The listing builds one solid part. Answer for the finished solid, in the listing's coordinates (mm). A direction names the side the tool comes from. Give positions to 0.01 mm unless a question says otherwise; leave off trailing zeros. Order: outer loops, then holes, each group sorted by start corner. A loop starts at its lowest first (then second) coordinate and runs counter-clockwise, first axis right, second up. Notation, with made-up numbers: (-4, 44) - (28, 44) arc R22 cw to (28, 76) - close; hole circle Ø11 at (-1.5, 73.5). An arc over 180 degrees is marked (long way). Answer in a Markdown table with one row per item.
from build123d import *

# Parameters (mm, degrees)
CROQUIS1_R              = 1.75
SALIENTE_EXTRUIR1_DEPTH = 3
CROQUIS3_W              = 6
CROQUIS3_H              = 30
CROQUIS3_R              = 1.75
SALIENTE_EXTRUIR4_DEPTH = 14
REDONDEO1_R             = 2


with BuildPart() as part:
    # Croquis1 → Saliente-Extruir1 (new body)
    # profile 1 of 2: a face of its own
    with BuildSketch(Plane.XY):
        Polygon((-24, 12.5), (24, 12.5), (24, 22.5), (24, 27.5), (-24, 27.5), (-24, 22.5), align=None)
        with Locations((-21, 25)):
            Circle(CROQUIS1_R, mode=Mode.SUBTRACT)
        with Locations((21, 25)):
            Circle(CROQUIS1_R, mode=Mode.SUBTRACT)
    # profile 2 of 2: a face of its own
    with BuildSketch(Plane.XY):
        Polygon((-24, -2.5), (24, -2.5), (24, 2.5), (24, 12.5), (-24, 12.5), (-24, 2.5), align=None)
        with Locations((-21, 0)):
            Circle(CROQUIS1_R, mode=Mode.SUBTRACT)
        with Locations((21, 0)):
            Circle(CROQUIS1_R, mode=Mode.SUBTRACT)
    extrude(amount=SALIENTE_EXTRUIR1_DEPTH)

    # Croquis3 → Saliente-Extruir4 (add)
    # profile 1 of 2: a face of its own
    with BuildSketch(Plane.XY.offset(3)):
        with Locations((-21, 12.5)):
            Rectangle(CROQUIS3_W, CROQUIS3_H)
        with Locations((-21, 0)):
            Circle(CROQUIS3_R, mode=Mode.SUBTRACT)
        with Locations((-21, 25)):
            Circle(CROQUIS3_R, mode=Mode.SUBTRACT)
    # profile 2 of 2: a face of its own
    with BuildSketch(Plane.XY.offset(3)):
        with Locations((21, 12.5)):
            Rectangle(CROQUIS3_W, CROQUIS3_H)
        with Locations((21, 0)):
            Circle(CROQUIS3_R, mode=Mode.SUBTRACT)
        with Locations((21, 25)):
            Circle(CROQUIS3_R, mode=Mode.SUBTRACT)
    extrude(amount=SALIENTE_EXTRUIR4_DEPTH)

    # Redondeo1
    # the kernel refuses this fillet: 2 mm, written as the material it takes off along each edge
    with BuildSketch(Plane(origin=(-24, 32.5, 0), x_dir=(1, 0, 0), z_dir=(0, -1, 0)), Plane(origin=(24, -7.5, 0), x_dir=(-1, 0, 0), z_dir=(0, 1, 0))) as redondeo1_piece_1:
        with BuildLine():
            CenterArc((REDONDEO1_R, REDONDEO1_R), REDONDEO1_R, 180, 90)
            Line((0, REDONDEO1_R), (0, 0))
            Line((0, 0), (REDONDEO1_R, 0))
        make_face()
    extrude(amount=40, mode=Mode.SUBTRACT)


solid = part.part
Item 1: Consider line 1 (X direction, y = 0, z = 5.25); line 2 (Y direction, x = 21, z = 12.25); line 3 (X direction, y = 5, z = 12.75). Determine where each line is inside the solid, lowest interval first.
Answer block:
| item | result |
|---|---|
| line 1 | -24 to -22.75, -19.25 to -18, 18 to 19.25, 22.75 to 24 |
| line 2 | -2.5 to -1.75, 1.75 to 23.25, 26.75 to 27.5 |
| line 3 | -24 to -18, 18 to 24 |
Item 2: Find section D-D on y = 19.5. Write down the section's boundary in (x, z), then the cut area to 3 significant figures.
Answer block:
| item | result |
|---|---|
| outline | (-24, 2) arc R2 ccw to (-22, 0) - (22, 0) arc R2 ccw to (24, 2) - (24, 17) - (18, 17) - (18, 3) - (-18, 3) - (-18, 17) - (-24, 17) - close |
| area | 310 mm² |
Item 3: Find section B-B on x = 21. Write down the section's boundary in (y, z).
Answer block:
| item | result |
|---|---|
| outline | (-2.5, 0) - (-1.75, 0) - (-1.75, 17) - (-2.5, 17) - close; (1.75, 0) - (23.25, 0) - (23.25, 17) - (1.75, 17) - close; (26.75, 0) - (27.5, 0) - (27.5, 17) - (26.75, 17) - close |
Item 4: Determine the mould class of faces 3 (the face through (-0.3, 27.5, 2.7)), 4 (the face through (23.43, 12.29, 0.6)), 5 (the face through (19.71, 26.18, 8.38)) for opening direction X: pulls with the +X half, pulls with the -X half, needs draft (parallel to the pull), parting line crosses it, or undercut.
Answer block:
| item | result |
|---|---|
| face 3 | needs draft |
| face 4 | pulls with the +X half |
| face 5 | undercut |
Item 5: This flat-tipped pin is pushed along its axis until it touches: P1, Ø3, axis at x = -21, y = 0, coming from the +Z side. Where does it stop, or does it pass through?
Answer block:
| item | result |
|---|---|
| P1 | through |
Item 6: Find section A-A on z = 12. Write down the section's boundary in (x, y).
Answer block:
| item | result |
|---|---|
| outline | (-24, -2.5) - (-18, -2.5) - (-18, 27.5) - (-24, 27.5) - close; (18, -2.5) - (24, -2.5) - (24, 27.5) - (18, 27.5) - close; hole circle Ø3.5 at (-21, 0); hole circle Ø3.5 at (-21, 25); hole circle Ø3.5 at (21, 0); hole circle Ø3.5 at (21, 25) |
Item 7: Find section C-C on y = 0. Write down the section's boundary in (x, z).
Answer block:
| item | result |
|---|---|
| outline | (-24, 2) arc R2 ccw to (-22.75, 0.15) - (-22.75, 17) - (-24, 17) - close; (-19.25, 0) - (19.25, 0) - (19.25, 17) - (18, 17) - (18, 3) - (-18, 3) - (-18, 17) - (-19.25, 17) - close; (22.75, 0.15) arc R2 ccw to (24, 2) - (24, 17) - (22.75, 17) - close |
Item 8: Which of the six approach directions +Z, -Z, +X, -X, +Y, -Y give full straight-line access (tool end or side, diameter ignored) to faces 1 (the face through (19.25, 0.08, 8.38)), 2 (the face through (18, 12, 10))?
Answer block:
| item | result |
|---|---|
| face 1 | +Z, -Z |
| face 2 | +Z, +Y, -Y |
